Can you work these out from the model? Positions are in its coordinate system, mm. Face numbers are marked on the shaded views. A direction names the side the tool comes from. Coordinates: 2 decimals unless noted, no trailing zeros. Loops run counter-clockwise (first coordinate to the right, second up) from the corner with the lowest first, then second, coordinate; pieces in that order, holes last. Notation, with made-up numbers: (28, 49) -> (84, 49) arc R9 ccw to (84, 62) -> close; hole circle Ø5 at (11.25, 61). An arc over 180 degrees is marked (long way). Put each result on its own line as item: value. Start each with the question number.
Item 1: If we section it at A-A on x = 8: Please give me the cut outline in (y, z), plus the area to 3 significant figures.
Item 2: For the marked faces 1, 2 and 3, which set-ups out of +Z, -Z, +X, -X, +Y, -Y let a thin tool reach every point of the face, with its end or its side?
Item 3: Please list where these lines run through material, in increasing order: L1, parallel to X at y = -13.6, z = 0; L2, parallel to Y at x = 6.5, z = -5; L3, parallel to Z at x = 8, y = -12.6. Write a range as from..to.
Item 4: Will these pins go through, and if not, where does the flat tip stop? P1, Ø3, axis at x = -8, z = -9, coming from the -Y side; P2, Ø4, axis at y = -16.5, z = -8.5, coming from the +X side; P3, Ø3, axis at x = -1.5, y = -23.5, coming from the -Z side.
Item 5: If we section it at B-B on z = -20: Please give me the cut outline in (x, y), plus the area to 3 significant figures.
Item 6: If we section it at D-D on x = -2.25: Please give me the cut outline in (y, z).
Item 7: If we section it at C-C on y = -23: Please give me the cut outline in (x, z).
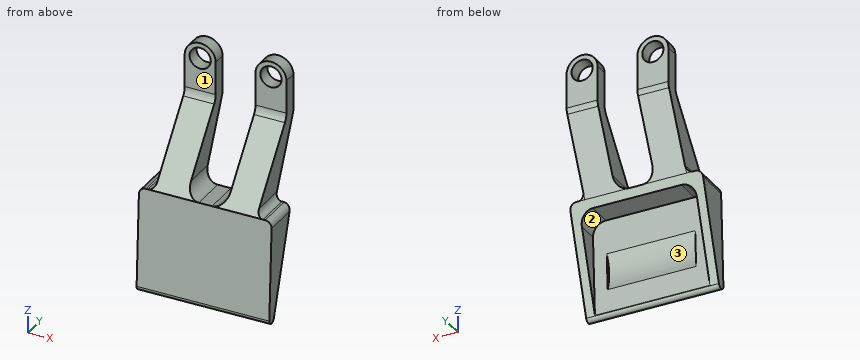
```python
from build123d import *

# Parameters (mm, degrees)
BOSS_EXTRUDE1_DEPTH   = 15
CUT_EXTRUDE1_REACH    = 66.15
SKETCH2_W             = 26
SKETCH2_H             = 30
SKETCH4_W             = 7
SKETCH4_H             = 12
SKETCH4_R             = 2.4
BOSS_EXTRUDE2_DEPTH   = 1.5
BOSS_EXTRUDE2_2_DEPTH = 1.5
BOSS_EXTRUDE3_DEPTH   = 7
BOSS_EXTRUDE4_DEPTH   = 7
FILLET1_R             = 3
FILLET2_R             = 1.5
FILLET3_R             = 1
FILLET4_RADIUS        = 3.5
FILLET4_LENGTH        = 3
FILLET5_RADIUS        = 3.5
FILLET5_LENGTH        = 3
SKETCH3_R             = 10
CUT_EXTRUDE2_DEPTH    = 10


with BuildPart() as part:
    # Sketch1 → Boss-Extrude1 (new, symmetric)
    with BuildSketch(Plane(origin=(0, 0, 0), x_dir=(0, 0, -1), z_dir=(1, 0, 0))):
        Polygon((25, -19.840542805), (25, -28), (55, -29.414764086), align=None)
    extrude(amount=BOSS_EXTRUDE1_DEPTH, both=True)

    # Cut-Extrude1: up to this plane
    cut_extrude1_end = Plane(origin=(0, -24.763733838, 1.167828043), z_dir=(0, -0.99888987496197, 0.0471064507096427))
    # Sketch2 → Cut-Extrude1 (cut, up to the surface)
    with BuildSketch(Plane(origin=(0, 0, 0), x_dir=(1, 0, 0), z_dir=(0, 1, 0)), mode=Mode.PRIVATE) as cut_extrude1_sk1:
        with Locations((0, 42)):
            Rectangle(SKETCH2_W, SKETCH2_H)
    cut_extrude1_tool1 = split(extrude(cut_extrude1_sk1.sketch, amount=-CUT_EXTRUDE1_REACH, mode=Mode.PRIVATE), bisect_by=cut_extrude1_end, keep=Keep.BOTH, mode=Mode.PRIVATE)
    add(cut_extrude1_tool1.solids().sort_by_distance((0, 0, -42))[0], mode=Mode.SUBTRACT)



with BuildPart() as body_2:
    # Sketch4 → Boss-Extrude2 (new, symmetric)
    with BuildSketch(Plane(origin=(0, -13.5, 0), x_dir=(1, 0, 0), z_dir=(0, 1, 0))):
        with Locations((8, 2.5)):
            Rectangle(SKETCH4_W, SKETCH4_H)
        with Locations(Location((8, 0, 0), (0, 0, 90))):
            Circle(SKETCH4_R, mode=Mode.SUBTRACT)
    extrude(amount=BOSS_EXTRUDE2_DEPTH, both=True)


with BuildPart() as body_3:
    # Sketch4 → Boss-Extrude2 2 (new, symmetric)
    with BuildSketch(Plane(origin=(0, -13.5, 0), x_dir=(1, 0, 0), z_dir=(0, 1, 0))):
        with Locations((-8, 2.5)):
            Rectangle(SKETCH4_W, SKETCH4_H)
        with Locations(Location((-8, 0, 0), (0, 0, 270))):
            Circle(SKETCH4_R, mode=Mode.SUBTRACT)
    extrude(amount=BOSS_EXTRUDE2_2_DEPTH, both=True)


with BuildPart() as part_1:
    add(part.part)

    add(body_2.part)  # Boss-Extrude3 merges body 2
    # Sketch5 → Boss-Extrude3 (add)
    with BuildSketch(Plane(origin=(11.5, 0, 0), x_dir=(0, 0, -1), z_dir=(1, 0, 0))):
        Polygon((8.5, -12), (8.5, -15), (25, -28), (25, -19.840542805), align=None)
    extrude(amount=-BOSS_EXTRUDE3_DEPTH)


    add(body_3.part)  # Boss-Extrude4 merges body 3
    # Sketch8 → Boss-Extrude4 (add)
    with BuildSketch(Plane.ZY.offset(11.5)):
        Polygon((-25, -28), (-8.5, -15), (-8.5, -12), (-25, -19.840542805), align=None)
    extrude(amount=-BOSS_EXTRUDE4_DEPTH)

    # Fillet1
    fillet1_edges = [part_1.edges().sort_by_distance(p)[0] for p in [
        (-8, -12, -8.5),
        (-4.5, -23.920271402, -25),
        (-13, -23.285459556, -27),
        (13, -23.285459556, -27),
        (8, -12, -8.5),
        (4.5, -23.920271402, -25),
        (8, -15, -8.5),
        (-8, -15, -8.5),
    ]]
    fillet(fillet1_edges, radius=FILLET1_R)

    # Fillet2
    # the kernel refuses this fillet: 1.5 mm, written as the material it adds along each edge
    with BuildSketch(Plane(origin=(-11.5, -16.090542805, -25), x_dir=(0, 0, 1), z_dir=(0, -1, 0))) as fillet2_piece_1_section:
        with BuildLine():
            CenterArc((FILLET2_R, FILLET2_R), FILLET2_R, 180, 90)
            Line((0, FILLET2_R), (0, 0))
            Line((0, 0), (FILLET2_R, 0))
        make_face()
    fillet2_piece_1 = extrude(amount=15.659457195, mode=Mode.PRIVATE)
    fillet2_piece_1 = split(fillet2_piece_1, bisect_by=Plane(origin=(-11.659708769, -19.629987495, -24.340243021), z_dir=(0, 0.9526614812535883, -0.30403306092548404)), keep=Keep.TOP, mode=Mode.PRIVATE)
    fillet2_piece_1 = split(fillet2_piece_1, bisect_by=Plane(origin=(-11.659708769, -19.543237279, -24.374336535), z_dir=(0, -0.9032129411473199, 0.4291927107302828)), keep=Keep.TOP, mode=Mode.PRIVATE)
    add(fillet2_piece_1)
    with BuildSketch(Plane(origin=(-11.5, -16.090542805, -25), x_dir=(0, 0, 1), z_dir=(0, -1, 0))) as fillet2_piece_2_section:
        with BuildLine():
            CenterArc((FILLET2_R, FILLET2_R), FILLET2_R, 180, 90)
            Line((0, FILLET2_R), (0, 0))
            Line((0, 0), (FILLET2_R, 0))
        make_face()
    fillet2_piece_2 = extrude(amount=15.659457195, mode=Mode.PRIVATE)
    fillet2_piece_2 = split(fillet2_piece_2, bisect_by=Plane(origin=(-11.843159529, -20.103961016, -25.825398338), z_dir=(0, -0.9526614812535883, 0.30403306092548404)), keep=Keep.TOP, mode=Mode.PRIVATE)
    fillet2_piece_2 = split(fillet2_piece_2, bisect_by=Plane(origin=(-11.843159529, -20.428696748, -26.237738291), z_dir=(0, -0.9032129411473199, 0.4291927107302828)), keep=Keep.TOP, mode=Mode.PRIVATE)
    fillet2_piece_2 = split(fillet2_piece_2, bisect_by=Plane(origin=(-11.843159529, -26.204484919, -22.721077013), z_dir=(0, 0.7854916722275349, -0.6188722266035137)), keep=Keep.TOP, mode=Mode.PRIVATE)
    fillet2_piece_2 = split(fillet2_piece_2, bisect_by=Plane(origin=(-11.843159529, -27.974843393, -24.466555432), z_dir=(0, 0.99888987496197, -0.04710645070964269)), keep=Keep.TOP, mode=Mode.PRIVATE)
    add(fillet2_piece_2)
    with BuildSketch(Plane(origin=(11.5, -31.75, -25), x_dir=(1, 0, 0), z_dir=(0, 1, 0))) as fillet2_piece_3_section:
        with BuildLine():
            CenterArc((FILLET2_R, -FILLET2_R), FILLET2_R, 90, 90)
            Line((0, -FILLET2_R), (0, 0))
            Line((0, 0), (FILLET2_R, 0))
        make_face()
    fillet2_piece_3 = extrude(amount=15.659457195, mode=Mode.PRIVATE)
    fillet2_piece_3 = split(fillet2_piece_3, bisect_by=Plane(origin=(11.843159529, -20.103961016, -25.825398338), z_dir=(0, -0.9526614812535883, 0.30403306092548404)), keep=Keep.TOP, mode=Mode.PRIVATE)
    fillet2_piece_3 = split(fillet2_piece_3, bisect_by=Plane(origin=(11.843159529, -27.974843393, -24.466555432), z_dir=(0, 0.99888987496197, -0.04710645070964269)), keep=Keep.TOP, mode=Mode.PRIVATE)
    fillet2_piece_3 = split(fillet2_piece_3, bisect_by=Plane(origin=(11.843159529, -26.204484919, -22.721077013), z_dir=(0, 0.7854916722275349, -0.6188722266035137)), keep=Keep.TOP, mode=Mode.PRIVATE)
    fillet2_piece_3 = split(fillet2_piece_3, bisect_by=Plane(origin=(11.843159529, -20.428696748, -26.237738291), z_dir=(0, -0.9032129411473199, 0.4291927107302828)), keep=Keep.TOP, mode=Mode.PRIVATE)
    add(fillet2_piece_3)
    with BuildSketch(Plane(origin=(11.5, -31.75, -25), x_dir=(1, 0, 0), z_dir=(0, 1, 0))) as fillet2_piece_4_section:
        with BuildLine():
            CenterArc((FILLET2_R, -FILLET2_R), FILLET2_R, 90, 90)
            Line((0, -FILLET2_R), (0, 0))
            Line((0, 0), (FILLET2_R, 0))
        make_face()
    fillet2_piece_4 = extrude(amount=15.659457195, mode=Mode.PRIVATE)
    fillet2_piece_4 = split(fillet2_piece_4, bisect_by=Plane(origin=(11.659708769, -19.629987495, -24.340243021), z_dir=(0, 0.9526614812535883, -0.30403306092548404)), keep=Keep.TOP, mode=Mode.PRIVATE)
    fillet2_piece_4 = split(fillet2_piece_4, bisect_by=Plane(origin=(11.659708769, -19.543237279, -24.374336535), z_dir=(0, -0.9032129411473199, 0.4291927107302828)), keep=Keep.TOP, mode=Mode.PRIVATE)
    add(fillet2_piece_4)
    # the kernel refuses this fillet: 1.5 mm, written as the material it takes off along each edge
    with BuildSketch(Plane(origin=(-15, -16.090542805, -25), x_dir=(1, 0, 0), z_dir=(0, -1, 0)), Plane(origin=(15, -16.090542805, -25), x_dir=(0, 0, -1), z_dir=(0, -1, 0))) as fillet2_2_piece_1:
        with BuildLine():
            CenterArc((FILLET2_R, -FILLET2_R), FILLET2_R, 90, 90)
            Line((0, -FILLET2_R), (0, 0))
            Line((0, 0), (FILLET2_R, 0))
        make_face()
    extrude(amount=15.659457195, mode=Mode.SUBTRACT)

    # Fillet3
    fillet3_edges = [part_1.edges().sort_by_distance(p)[0] for p in [
        (0, -29.414764086, -55),
    ]]
    fillet(fillet3_edges, radius=FILLET3_R)

    # Fillet4: full round fillet: the end face becomes a half cylinder, R = half its width
    fillet4_face = Plane((8, -13.5, 3.5), x_dir=(0, 1, 0), z_dir=(0, 0, 1))  # on the end face: x along it, z out of the body
    fillet4_slab = fillet4_face.offset(-FILLET4_RADIUS / 2) * Box(FILLET4_LENGTH, 2 * FILLET4_RADIUS, FILLET4_RADIUS, mode=Mode.PRIVATE)  # the body's end, R deep
    fillet4_round = Plane((8, -13.5, 0), x_dir=(0, 0, 1), z_dir=(0, 1, 0)) * Cylinder(FILLET4_RADIUS, FILLET4_LENGTH, mode=Mode.PRIVATE)  # its axis R under the face
    add(fillet4_slab - fillet4_round, mode=Mode.SUBTRACT)

    # Fillet5: full round fillet: the end face becomes a half cylinder, R = half its width
    fillet5_face = Plane((-8, -13.5, 3.5), x_dir=(0, 1, 0), z_dir=(0, 0, 1))  # on the end face: x along it, z out of the body
    fillet5_slab = fillet5_face.offset(-FILLET5_RADIUS / 2) * Box(FILLET5_LENGTH, 2 * FILLET5_RADIUS, FILLET5_RADIUS, mode=Mode.PRIVATE)  # the body's end, R deep
    fillet5_round = Plane((-8, -13.5, 0), x_dir=(0, 0, 1), z_dir=(0, 1, 0)) * Cylinder(FILLET5_RADIUS, FILLET5_LENGTH, mode=Mode.PRIVATE)  # its axis R under the face
    add(fillet5_slab - fillet5_round, mode=Mode.SUBTRACT)

    # Sketch3 → Cut-Extrude2 (cut, symmetric)
    with BuildSketch(Plane(origin=(0, 0, 0), x_dir=(0, 0, -1), z_dir=(1, 0, 0))):
        with Locations((39, -17.5)):
            Circle(SKETCH3_R)
    extrude(amount=CUT_EXTRUDE2_DEPTH, both=True, mode=Mode.SUBTRACT)


solid = part_1.part
```
Solutions:
1. outline: (-29.06, -47.41) arc R1 ccw to (-27.11, -47.76) -> (-27.07, -47.64) -> (-26.83, -42.6) arc R10 cw to (-26.45, -34.53) -> (-26.09, -27) -> (-20.48, -27) -> (-19.84, -25) -> (-12.29, -9.11) arc R3 ccw to (-12, -7.82) -> (-12, -2.4) -> (-15, -2.4) -> (-15, -7.46) arc R3 cw to (-15.64, -9.32) -> (-28, -25) -> close; (-15, 2.4) -> (-12, 2.4) -> (-12, 3.5) -> (-15, 3.5) -> close
1. area: 167 mm^2
2. face 1: +Z, +X, -X, -Y
2. face 2: -Z, +Y
2. face 3: +Y
3. L1: -11.5..-10.4, -5.6..-4.5, 4.5..5.6, 10.4..11.5
3. L2: -15..-12
3. L3: -9.76..-2.4, 2.4..3.5
4. P1: y = -16.58
4. P2: x = 11.5
4. P3: z = -27
5. outline: (-11.5, -24.06) -> (-4.5, -24.06) -> (-4.5, -17.46) -> (-11.5, -17.46) -> close; (4.5, -24.06) -> (11.5, -24.06) -> (11.5, -17.46) -> (4.5, -17.46) -> close
5. area: 92.3 mm^2
6. outline: (-29.06, -47.41) arc R1 ccw to (-27.11, -47.76) -> (-27.07, -47.64) -> (-26.83, -42.6) arc R10 cw to (-26.45, -34.53) -> (-26.09, -27) -> (-20.48, -27) -> (-19.84, -25) -> (-19.8, -24.9) -> (-27.92, -24.9) -> (-28, -25) -> close
7. outline: (-15, -34.9) -> (-13, -34.9) -> (-13, -30) arc R3 cw to (-10, -27) -> (10, -27) arc R3 cw to (13, -30) -> (13, -34.9) -> (15, -34.9) -> (15, -26.5) arc R1.5 ccw to (13.5, -25) -> (13, -25) arc R1.5 cw to (11.5, -23.5) -> (11.5, -18.65) -> (4.5, -18.65) -> (4.5, -22) arc R3 cw to (1.5, -25) -> (-1.5, -25) arc R3 cw to (-4.5, -22) -> (-4.5, -18.65) -> (-11.5, -18.65) -> (-11.5, -23.5) arc R1.5 cw to (-13, -25) -> (-13.5, -25) arc R1.5 ccw to (-15, -26.5) -> close
